from build123d import *

# Parameters (mm, degrees)
SKETCH2_R           = 9.525
BOSS_EXTRUDE1_DEPTH = 237.399999964
SKETCH3_R           = 8.621005773
BOSS_EXTRUDE2_DEPTH = 12.7
SKETCH4_R           = 7.9375
BOSS_EXTRUDE3_DEPTH = 12.7


with BuildPart() as part:
    # Sketch2 → Boss-Extrude1 (new body)
    with BuildSketch(Plane(origin=(0, 0, 0), x_dir=(1, 0, 0), z_dir=(0, 1, 0))):
        Circle(SKETCH2_R)
    extrude(amount=BOSS_EXTRUDE1_DEPTH)

    # Sketch3 → Boss-Extrude2 (add)
    with BuildSketch(Plane(origin=(0, 237.399999964, 0), x_dir=(1, 0, 0), z_dir=(0, 1, 0))):
        Circle(SKETCH3_R)
    extrude(amount=BOSS_EXTRUDE2_DEPTH)

    # Sketch4 → Boss-Extrude3 (add)
    with BuildSketch(Plane.XZ):
        Circle(SKETCH4_R)
    extrude(amount=BOSS_EXTRUDE3_DEPTH)


solid = part.part
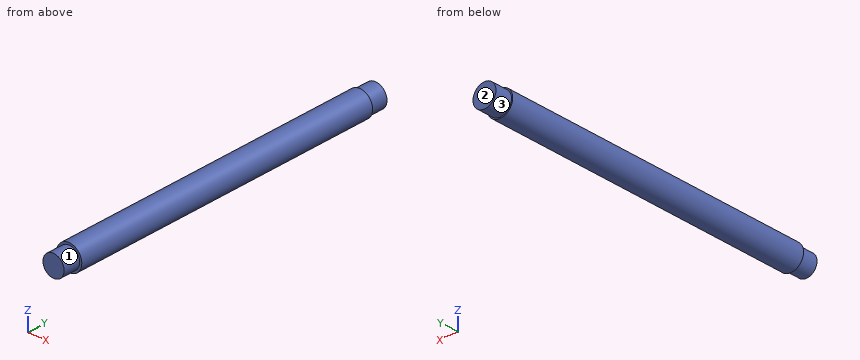
Input: part model. Units: mm. Frame: model coordinates. Face numbers are marked on the shaded views. A direction names the side the tool comes from. Coordinates: 2 decimals unless noted, no trailing zeros. Loops run counter-clockwise (first coordinate to the right, second up) from the corner with the lowest first, then second, coordinate; pieces in that order, holes last. Notation, with made-up numbers: (57, 5) - (104, 5) arc R24 cw to (104, 20) - close; hole circle Ø2 at (58.5, 50). An arc over 180 degrees is marked (long way). Answer in a Markdown table with one row per item. Add a question column.
Item 1: Access query for the marked faces 1, 2 and 3. Directions: +Z, -Z, +X, -X, +Y, -Y. A direction counts if a zero-diameter tool reaches every point of the face in a straight line with its end or side. Return the directions, or none.
Item 2: Contact query for flat-ended pins moving along their axis: P1, Ø2, axis at y = 26.5, z = -1.5, coming from the -X side; P2, Ø6, axis at x = -3.5, y = 114.5, coming from the -Z side; P3, Ø2, axis at x = -7, y = 110.5, coming from the +Z side. Output: stop coordinate, or through.
Item 3: Line query: line 1 along Z through (x, y) = (0.5, 197); line 2 along Y through (x, z) = (7.75, -4.5). Output: solid intervals per line, ascending. Write a range as [from, to].
Item 4: Section query B-B on x = 4.75. Return the cut outline in (y, z), then the cut area to 3 significant figures.
Item 5: Section query A-A on z = -3.25. Return the cut outline in (x, y), then the cut area to 3 significant figures.
Item 6: Section query C-C on y = 162. Return the cut outline in (x, z) (3 decimals), then the cut area to 3 significant figures.
Recorded:
| question | item | result |
|---|---|---|
| 1 | face 1 | -Y |
| 1 | face 2 | +Z, -Z, +X, -X, +Y |
| 1 | face 3 | +Y |
| 2 | P1 | x = -9.51 |
| 2 | P2 | z = -9.51 |
| 2 | P3 | z = 7.4 |
| 3 | line 1 | [-9.51, 9.51] |
| 3 | line 2 | [0, 237.4] |
| 4 | outline | (-12.7, -6.36) - (0, -6.36) - (0, -8.26) - (237.4, -8.26) - (237.4, -7.19) - (250.1, -7.19) - (250.1, 7.19) - (237.4, 7.19) - (237.4, 8.26) - (0, 8.26) - (0, 6.36) - (-12.7, 6.36) - close |
| 4 | area | 4,260 mm^2 |
| 5 | outline | (-8.95, 0) - (-7.24, 0) - (-7.24, -12.7) - (7.24, -12.7) - (7.24, 0) - (8.95, 0) - (8.95, 237.4) - (7.98, 237.4) - (7.98, 250.1) - (-7.98, 250.1) - (-7.98, 237.4) - (-8.95, 237.4) - close |
| 5 | area | 4,640 mm^2 |
| 6 | outline | circle Ø19.05 at (0, 0) |
| 6 | area | 285 mm^2 |
